CAD build for the part. Positions are in the model's coordinates, mm. Face numbers are marked on the shaded views. A direction names the side the tool comes from. Coordinates: 2 decimals unless noted, no trailing zeros. Loops run counter-clockwise (first coordinate to the right, second up) from the corner with the lowest first, then second, coordinate; pieces in that order, holes last. Notation, with made-up numbers: (71.5, -17) -> (86.5, -17) arc R19 cw to (86.5, 20) -> close; hole circle Ø2 at (-30, 44.25). An arc over 180 degrees is marked (long way). Write each question's results on one line, items separated by ' | '.
Autodesk Inventor part; units mm, degrees
ref_plane "YZ Plane" through (0, 0, 0) normal (1, 0, 0) x (0, 1, 0)
ref_plane "XZ Plane" through (0, 0, 0) normal (0, 1, 0) x (-1, 0, 0)
ref_plane "XY Plane" through (0, 0, 0) normal (0, 0, 1) x (1, 0, 0)
sketch "Sketch1" plane through (0, 0, 0) normal (1, 0, 0) x (0, 1, 0)
  line L0 (13.9123, 0.5821) -> (-10.2877, 0.5821)
  line L1 (-10.6877, 0.1821) -> (-10.6877, -2.0179)
  line L2 (-10.2877, -2.4179) -> (13.9123, -2.4179)
  line L3 (14.3123, -2.0179) -> (14.3123, 0.1821)
  arc A0 (13.9123, -2.4179) -> (14.3123, -2.0179) centre (13.9123, -2.0179) ccw
  arc A1 (14.3123, 0.1821) -> (13.9123, 0.5821) centre (13.9123, 0.1821) ccw
  arc A2 (-10.6877, -2.0179) -> (-10.2877, -2.4179) centre (-10.2877, -2.0179) ccw
  arc A3 (-10.2877, 0.5821) -> (-10.6877, 0.1821) centre (-10.2877, 0.1821) ccw
  line L4 (14.3123, -4.8123) -> (1.8123, -4.8123) construction
  line L5 (14.3123, 0.1821) -> (14.3123, -23.1695) construction
  circle A4 centre (1.8123, -0.9179) radius 3
  circle A5 centre (1.8123, -0.9179) radius 1.5
  point P0 (0, 0)
  point P1 (-10.6877, -2.4179)
  point P2 (-10.6877, 0.5821)
  point P3 (14.3123, -2.4179)
  point P4 (4.4103, 0.5821)
  point P5 (-0.7858, 0.5821)
  point P6 (-0.7858, -2.4179)
  point P7 (4.4103, -2.4179)
  dimension "d1" = 3
  dimension "d2" = 25
  dimension "d3" = 0.4
  dimension "d4" = 12.5
  dimension "d5" = 6
extrude "Extrusion1" add sketch "Sketch1" along normal blind 2
extrude "Extrusion2" add sketch "Sketch1" against normal blind 2 contours A4 L2 A5 L0 | L0 A4 | A5 L2 A4 L0 | A5 | L2 A4
extrude "Extrusion3" add sketch "Sketch1" against normal blind 3 contours A5
fillet "Fillet1" radius 0.5 1 edges at (-3, 0.3123, -0.9179)
fillet "Fillet2" radius 0.5 1 edges at (-2, -1.1877, -0.9179)
fillet "Fillet3" radius 0.5 10 edges at (0, 14.1951, 0.465) (0, 14.3123, -0.9179) (0, 14.1951, -2.3007) (0, 9.1613, -2.4179) (0, 9.1613, 0.5821) (0, -10.5706, 0.465) (0, -10.6877, -0.9179) (0, -10.5706, -2.3007) (0, -5.5368, -2.4179) (0, -5.5368, 0.5821)
sketch "Sketch2" plane through (2, 0, 0) normal (1, 0, 0) x (0, 0, -1)
  line L0 (-0.5821, 13.9123) -> (-0.5821, 4.4103)
  arc A0 (-0.5821, 4.4103) -> (-0.5821, -0.7858) centre (0.9179, 1.8123) ccw
  line L1 (-0.5821, -0.7858) -> (-0.5821, -10.2877)
  arc A1 (-0.5821, -10.2877) -> (-0.1821, -10.6877) centre (-0.1821, -10.2877) ccw
  line L2 (-0.1821, -10.6877) -> (2.0179, -10.6877)
  arc A2 (2.0179, -10.6877) -> (2.4179, -10.2877) centre (2.0179, -10.2877) ccw
  line L3 (2.4179, -10.2877) -> (2.4179, -0.7858)
  arc A3 (2.4179, -0.7858) -> (2.4179, 4.4103) centre (0.9179, 1.8123) ccw
  line L4 (2.4179, 4.4103) -> (2.4179, 13.9123)
  arc A4 (2.4179, 13.9123) -> (2.0179, 14.3123) centre (2.0179, 13.9123) ccw
  line L5 (2.0179, 14.3123) -> (-0.1821, 14.3123)
  arc A5 (-0.1821, 14.3123) -> (-0.5821, 13.9123) centre (-0.1821, 13.9123) ccw
  point P0 (0, 0)
extrude "Extrusion4" add sketch "Sketch2" along normal blind 3
properties part number "torque"
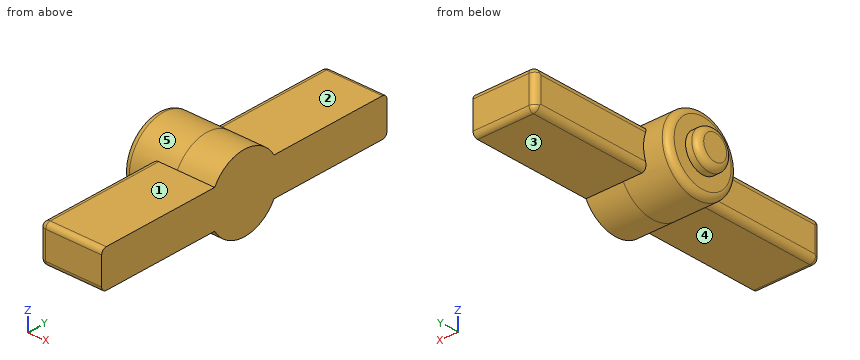
1) Pin check, flat tips, straight feed: pin 1 (2 mm diameter, centred on x = 4, y = 8, fed in from -Z); pin 2 (1.3 mm diameter, centred on x = 3.5, y = -5.5, fed in from +Z); pin 3 (1.6 mm diameter, centred on y = 11.5, z = -0.5, fed in from -X). Stop position of each tip, or through.
Outcome:
pin 1: stops at z = -2.42 | pin 2: stops at z = 0.58 | pin 3: stops at x = 0
2) Slice it at C-C (x = -0.5). Write the cut outline in (y, z), then the cut area to 3 significant figures.
Outcome:
outline: circle Ø6 at (1.81, -0.92) | area: 28.3 mm^2
3) Drill centre lines: L1, parallel to X at y = 6.5, z = -0.5; L2, parallel to X at y = 1.75, z = -2.75; L3, parallel to Z at x = 4.75, y = 6. Where is each one in solid material? Low to high. Write a range as from..to.
Outcome:
L1: x = 0..5 | L2: x = -2..5 | L3: z = -2.42..0.58
4) Slice it at A-A (y = 8.25). Write the cut outline in (x, z), then the cut area to 3 significant figures.
Outcome:
outline: (0, -1.92) arc R0.5 ccw to (0.5, -2.42) -> (5, -2.42) -> (5, 0.58) -> (0.5, 0.58) arc R0.5 ccw to (0, 0.08) -> close | area: 14.9 mm^2
5) Slice it at B-B (x = 2.25). Write the cut outline in (y, z), then the cut area to 3 significant figures.
Outcome:
outline: (-10.69, -2.02) arc R0.4 ccw to (-10.29, -2.42) -> (-0.79, -2.42) arc R3 ccw to (4.41, -2.42) -> (13.91, -2.42) arc R0.4 ccw to (14.31, -2.02) -> (14.31, 0.18) arc R0.4 ccw to (13.91, 0.58) -> (4.41, 0.58) arc R3 ccw to (-0.79, 0.58) -> (-10.29, 0.58) arc R0.4 ccw to (-10.69, 0.18) -> close | area: 85.9 mm^2
6) Which spindle directions (+Z, -Z, +X, -X, +Y, -Y) get a long thin tool onto all of the face, cutting with end or side? Do the marked faces 1, 2, 3, 4 and 5. Say none if no direction does.
Outcome:
face 1: +Z, +X, -X, -Y | face 2: +Z, +X, -X, +Y | face 3: -Z, +X, -X, +Y | face 4: -Z, +X, -X, -Y | face 5: -X
